Design review of the part shown in the three views and the two pictorial views. Dimensions are in mm from the part's minimum x, y and z. Round coordinates to 2 decimals unless told otherwise and drop trailing zeros. Write each loop counter-clockwise with the first axis right and the second up, starting at its lowest first coordinate (ties: lowest second). Pieces come first, ordered by that corner, then holes. Notation, with made-up numbers: (26.5, 63) - (80.5, 63) arc R20 ccw to (80.5, 78) - close; hole circle Ø10 at (54.25, 89.25). An arc over 180 degrees is marked (long way). Use one line per item in the form item = value.
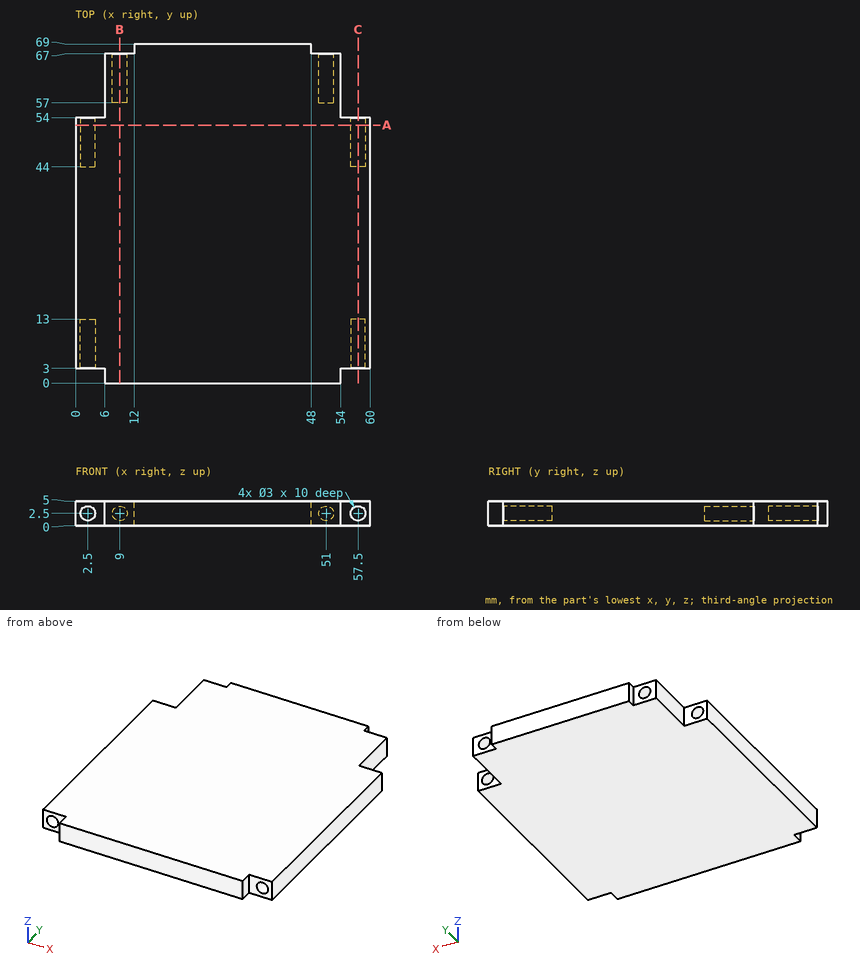
Q1. We need section B-B on x = 9. Write out the cut boundary in (y, z).
Calculated:
outline = (0, 0) - (67, 0) - (67, 1) - (57, 1) - (57, 4) - (67, 4) - (67, 5) - (0, 5) - close
Q2. We need section A-A on y = 52.5. Write out the cut boundary in (x, z).
Calculated:
outline = (0, 0) - (60, 0) - (60, 5) - (0, 5) - close; hole circle Ø3 at (2.5, 2.5); hole circle Ø3 at (57.5, 2.5)
Q3. We need section C-C on x = 57.5. Write out the cut boundary in (y, z), then the cut area to 3 significant figures.
Calculated:
outline = (3, 0) - (54, 0) - (54, 1) - (44, 1) - (44, 4) - (54, 4) - (54, 5) - (3, 5) - (3, 4) - (13, 4) - (13, 1) - (3, 1) - close
area = 195 mm2
Q4. For P1, Ø1.5, axis at x = 50, z = 1.5, coming from the +Y side; P2, Ø0.9, axis at x = 3, z = 3, coming from the -Y side; P3, Ø2.5, axis at y = 1.5, z = 1.5, coming from the -X side, all flat-tipped, find the tip position at first contact; note any pin that passes through.
Calculated:
P1 = 67
P2 = 13
P3 = 6
Q5. To check wall thickness, follow line 1 along Z through (x, y) = (2.5, 6.5); line 2 along Y through (x, z) = (50.5, 2.4); line 3 along X through (y, z) = (56.5, 2.7). State the ranges of each line that lie inside material, in increasing order. Write a range as from..to.
Calculated:
line_1 = 0..1, 4..5
line_2 = 0..57
line_3 = 6..54
